Autodesk Inventor part; units mm, degrees
ref_plane "YZ Plane" through (0, 0, 0) normal (1, 0, 0) x (0, 1, 0)
ref_plane "XZ Plane" through (0, 0, 0) normal (0, 1, 0) x (-1, 0, 0)
ref_plane "XY Plane" through (0, 0, 0) normal (0, 0, 1) x (1, 0, 0)
sketch "スケッチ1" plane through (0, 0, 0) normal (0, 1, 0) x (-1, 0, 0)
  line L0 (0, 0) -> (65.5, 0)
  line L1 (65.5, 0) -> (65.5, -70)
  line L2 (65.5, -70) -> (0, -70)
  line L3 (0, -70) -> (0, 0)
  dimension "d0" = 65.5
  dimension "d1" = 70
extrude "押し出し1" add sketch "スケッチ1" along normal blind 3
sketch "スケッチ2" plane through (0, 3, 0) normal (0, 1, 0) x (1, 0, 0)
  line L0 (-60.5, 5) -> (-5, 5)
  line L1 (-5, 5) -> (-5, 65)
  line L2 (-5, 65) -> (-60.5, 65)
  line L3 (-60.5, 65) -> (-60.5, 5)
  line L4 (-65.5, 0) -> (0, 0)
  line L5 (-65.5, 70) -> (-65.5, 0)
  dimension "d4" = 55.5
  dimension "d5" = 60
  dimension "d6" = 5
  dimension "d7" = 5
hole "穴1" at (-60.5, 3, -5) at (-5, 3, -5) at (-60.5, 3, -65) at (-5, 3, -65) direction (0, -1, 0) diameter 3.2 end through all
sketch "スケッチ3" plane through (0, 3, 0) normal (0, 1, 0) x (1, 0, 0)
  line L0 (-65.5, 0) -> (0, 0)
  line L1 (-32.75, 0) -> (-32.75, 70)
  line L2 (0, 70) -> (-65.5, 70)
  circle A0 centre (-32.75, 35) radius 15.18
  line L3 (0, 70) -> (-65.5, 70)
  line L4 (-65.5, 70) -> (-65.5, 0)
  point P0 (-32.75, 50.18)
  point P1 (-45.8963, 42.59)
  point P2 (-45.8963, 27.41)
  point P3 (-32.75, 19.82)
  point P4 (-19.6037, 27.41)
  point P5 (-19.6037, 42.59)
  dimension "d15" = 30.36
  dimension "d18" = 360
  dimension "d27" = 32.75
hole "穴2" at (-32.75, 3, -50.18) at (-45.8963, 3, -42.59) at (-45.8963, 3, -27.41) at (-32.75, 3, -19.82) at (-19.6037, 3, -27.41) at (-19.6037, 3, -42.59) direction (0, -1, 0) diameter 4.2 end through all
properties part number "link2_plate4" material "アルミニウム 6061"
Design review of the part built by this model. Coordinates are the model's own, in mm. Coordinates: 2 decimals unless noted, no trailing zeros. Order: outer loops, then holes, each group sorted by start corner. A loop starts at its lowest first (then second) coordinate and runs counter-clockwise, first axis right, second up. Notation, with made-up numbers: M 82,86.25 L 120,86.25 A20 cw 120,117.25 Z; hole C -30,80.25 d10. An arc over 180 degrees is marked long. Use a Markdown table: item, result.
(1) Add section A-A (z = -19.82). Give the boundary of the cut face in (x, y).
Worked answers:
| item | result |
|---|---|
| outline | M -65.5,0 L -34.85,0 L -34.85,3 L -65.5,3 Z; M -30.65,0 L 0,0 L 0,3 L -30.65,3 Z |
(2) Add section C-C (z = -42.59). Give the boundary of the cut face in (x, y), then the cut area to 3 significant figures.
Worked answers:
| item | result |
|---|---|
| outline | M -65.5,0 L -48,0 L -48,3 L -65.5,3 Z; M -43.8,0 L -21.7,0 L -21.7,3 L -43.8,3 Z; M -17.5,0 L 0,0 L 0,3 L -17.5,3 Z |
| area | 171 mm2 |
(3) Add section D-D (y = 1.75). Count the separate pieces of the cut face and the enclosed holes in it, then the cut area to 3 significant figures.
Worked answers:
| item | result |
|---|---|
| separate pieces | 1 |
| enclosed holes | 10 |
| area | 4,470 mm2 |
(4) Draft analysis for pull direction Z (two halves, no side actions). For faces 1 (the cylindrical face through (-61.85, 1.48, -64.14)), 2 (the flat face through (-33, 1, -70)), 3 (the flat face through (0, 1, -35)), 4 (the cylindrical face through (-4.03, 1.48, -6.27)), state which applies: released by +Z, released by -Z, zero draft, split by the parting line, or undercut.
Worked answers:
| item | result |
|---|---|
| face 1 | undercut |
| face 2 | released by -Z |
| face 3 | zero draft |
| face 4 | undercut |
(5) Wall thickness on probe 1 along Z at (x, y) = (-5, 1.45); probe 2 along X at (y, z) = (1.2, -5); probe 3 along X at (y, z) = (0.7, -43): over which ranges is each line inside the solid? List them lowest first.
Worked answers:
| item | result |
|---|---|
| probe 1 | z = -70 to -66.6, -63.4 to -6.6, -3.4 to 0 |
| probe 2 | x = -65.5 to -62.1, -58.9 to -6.6, -3.4 to 0 |
| probe 3 | x = -65.5 to -47.96, -43.84 to -21.66, -17.54 to 0 |
(6) Add section B-B (x = -32.75). Give the boundary of the cut face in (y, z), then the cut area to 3 significant figures.
Worked answers:
| item | result |
|---|---|
| outline | M 0,-70 L 3,-70 L 3,-52.28 L 0,-52.28 Z; M 0,-48.08 L 3,-48.08 L 3,-21.92 L 0,-21.92 Z; M 0,-17.72 L 3,-17.72 L 3,0 L 0,0 Z |
| area | 185 mm2 |
